The listing builds one solid part. Answer for the finished solid, in the listing's coordinates (mm). A direction names the side the tool comes from. Give positions to 0.01 mm unless a question says otherwise; leave off trailing zeros. Order: outer loops, then holes, each group sorted by start corner. A loop starts at its lowest first (then second) coordinate and runs counter-clockwise, first axis right, second up.
```python
from build123d import *

# Parameters (mm, degrees)
SKETCH_1_W      = 40
SKETCH_1_H      = 51.65
EXTRUDE_1_DEPTH = 12
SHELL_1_T       = -2
SKETCH_3_W      = 3.9
SKETCH_3_H      = 21.85
SKETCH_3_W_2    = 4.4
SKETCH_3_H_2    = 2
EXTRUDE_6_DEPTH = 10


with BuildPart() as part:
    # 草图1 → 凸台-拉伸1 (new body)
    with BuildSketch(Plane(origin=(0, 0, 0), x_dir=(0, 0, -1), z_dir=(1, 0, 0))):
        Rectangle(SKETCH_1_W, SKETCH_1_H)
    extrude(amount=EXTRUDE_1_DEPTH)

    # 抽壳1
    shell_1_openings = [part.faces().sort_by_distance(p)[0] for p in [
        (12, 0, 0),
    ]]
    offset(amount=SHELL_1_T, openings=shell_1_openings, kind=Kind.INTERSECTION)

    # 草图3 → 凸台-拉伸6 (add)
    # profile 1 of 2: a face of its own
    with BuildSketch(Plane(origin=(2, 0, 0), x_dir=(0, 0, -1), z_dir=(1, 0, 0))):
        Polygon((-2.9, 17.325), (3, 17.325), (3, 23.825), (5, 23.825), (5, 17.175), (5, -8.525), (-2.9, -8.525), (-2.9, -5.575), (-7.4, -5.575), (-7.4, -3.575), (-2.9, -3.575), align=None)
        with Locations((1.05, 4.4)):
            Rectangle(SKETCH_3_W, SKETCH_3_H, mode=Mode.SUBTRACT)
    # profile 2 of 2: a face of its own
    with BuildSketch(Plane(origin=(2, 0, 0), x_dir=(0, 0, -1), z_dir=(1, 0, 0))):
        with Locations((-15.8, -4.575)):
            Rectangle(SKETCH_3_W_2, SKETCH_3_H_2)
    extrude(amount=EXTRUDE_6_DEPTH)


solid = part.part
```
1) Find section C-C (z = -11). Write down the section's boundary in (x, y) (3 decimals).
Geometry says:
outline: (0, -25.825) - (12, -25.825) - (12, -23.825) - (2, -23.825) - (2, 23.825) - (12, 23.825) - (12, 25.825) - (0, 25.825) - close
2) Find section B-B (y = 9.5). Write down the section's boundary in (x, z).
Geometry says:
outline: (0, -20) - (12, -20) - (12, -18) - (2, -18) - (2, -5) - (12, -5) - (12, -3) - (2, -3) - (2, 0.9) - (12, 0.9) - (12, 2.9) - (2, 2.9) - (2, 18) - (12, 18) - (12, 20) - (0, 20) - close
3) Find section D-D (y = -14). Write down the section's boundary in (x, z).
Geometry says:
outline: (0, -20) - (12, -20) - (12, -18) - (2, -18) - (2, 18) - (12, 18) - (12, 20) - (0, 20) - close
4) Given P1, Ø4.5, axis at y = 3.5, z = -2, coming from the +X side, flat-ended and moving along its own axis, determine where the tip first touches the part or whether it passes through.
Geometry says:
P1: stops at x = 12
5) For a pull along Z with two mould halves and no side action, classify faces 3 (the flat face through (6, 0, 20)), 4 (the flat face through (7, -5.575, 5)), 5 (the flat face through (0, 0, 0)) as +Z half, -Z half, draft (parallel to the pull), parting line (faces both ways), or undercut.
Geometry says:
face 3: +Z half
face 4: undercut
face 5: draft
6) A tool of negligible diameter and unlimited length cuts with its end or side. For faces 1 (the flat face through (7, 4, -3)), 2 (the flat face through (12, 2, 2)), from which of +Z, -Z, +X, -X, +Y, -Y can it reach the whole face along a straight path? Write none if from no direction.
Geometry says:
face 1: +X
face 2: +Z, -Z, +X, +Y, -Y
7) Straight lines are drawn through the part: probe 1 along Z at (x, y) = (8.25, -6); probe 2 along Z at (x, y) = (3.25, 16); probe 3 along Z at (x, y) = (4, -4.5). For each, find the intervals that lie inside material, in ascending order.
Geometry says:
probe 1: z = -20 to -18, -5 to -3, 0.9 to 2.9, 18 to 20
probe 2: z = -20 to -18, -5 to 2.9, 18 to 20
probe 3: z = -20 to -18, -5 to -3, 0.9 to 7.4, 13.6 to 20
8) Find section A-A (x = 4.5). Write down the section's boundary in (y, z) (3 decimals), then the cut area to 3 significant figures.
Geometry says:
outline: (-25.825, -20) - (25.825, -20) - (25.825, 20) - (-25.825, 20) - close; hole (-23.825, -18) - (23.825, -18) - (23.825, -5) - (-8.525, -5) - (-8.525, 2.9) - (-5.575, 2.9) - (-5.575, 7.4) - (-3.575, 7.4) - (-3.575, 2.9) - (17.325, 2.9) - (17.325, -3) - (23.825, -3) - (23.825, 18) - (-3.575, 18) - (-3.575, 13.6) - (-5.575, 13.6) - (-5.575, 18) - (-23.825, 18) - close; hole (-6.525, -3) - (15.325, -3) - (15.325, 0.9) - (-6.525, 0.9) - close
area: 500 mm2
